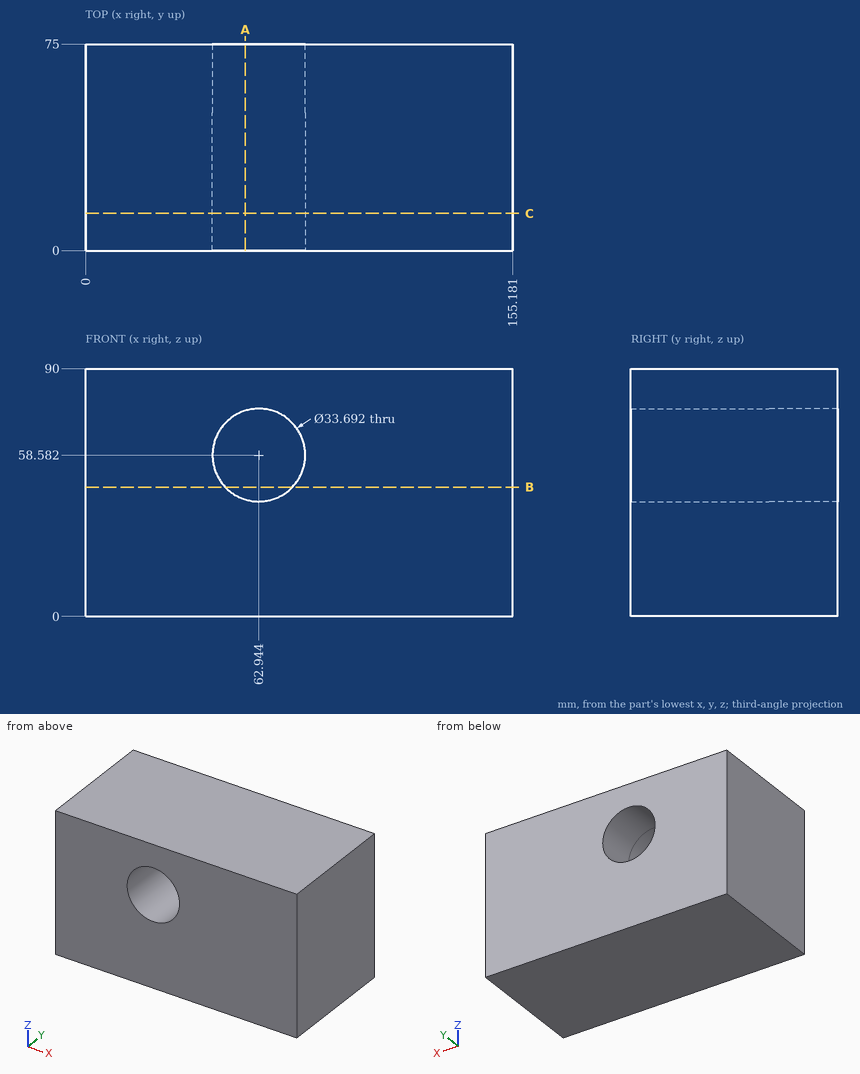
Source: three-view drawing plus pictorial views. Frame: mm from the lowest corner of the part. Give positions to 0.01 mm unless a question says otherwise; leave off trailing zeros. Order: outer loops, then holes, each group sorted by start corner. A loop starts at its lowest first (then second) coordinate and runs counter-clockwise, first axis right, second up.
1. Section A-A on x = 58. Return the cut outline in (y, z).
Derived:
outline: (0, 0) - (75, 0) - (75, 42.48) - (0, 42.48) - close; (0, 74.69) - (75, 74.69) - (75, 90) - (0, 90) - close
2. Section B-B on z = 47. Return the cut outline in (x, y), and give its area (3 significant figures).
Derived:
outline: (0, 0) - (50.71, 0) - (50.71, 75) - (0, 75) - close; (75.18, 0) - (155.18, 0) - (155.18, 75) - (75.18, 75) - close
area: 9,800 mm2
3. Material intervals for L1, parallel to X at y = 11, z = 62; L2, parallel to Z at x = 48.5, y = 6.5; L3, parallel to X at y = 12, z = 52, sorted ascending.
Derived:
L1: x = 0 to 46.45, 79.44 to 155.18
L2: z = 0 to 49.91, 67.25 to 90
L3: x = 0 to 47.44, 78.45 to 155.18
4. Section C-C on y = 13.5. Return the cut outline in (x, z).
Derived:
outline: (0, 0) - (155.18, 0) - (155.18, 90) - (0, 90) - close; hole circle Ø33.69 at (62.94, 58.58)
5. Pin query (flat end, axial travel): pin 1 (20 mm diameter, centred on x = 62.94, z = 58.58, fed in from -Y). Return the tip coordinate at first contact, or that it passes through.
Derived:
pin 1: passes through
